```python
from build123d import *

# Parameters (mm, degrees)
SKETCH_8_R               = 2.25
EXTRUDE_23_DEPTH         = 6.3
EXTRUDE_24_DEPTH         = 3.8
CUT_EXTRUDE_START        = -2
SKETCH_8_5_R             = 1
CUT_EXTRUDE_2_DEPTH      = 9.8
PATTERN_CIRCULAR_1_COUNT = 3
CUT_EXTRUDE_3_DEPTH      = 3.7
PATTERN_CIRCULAR_2_COUNT = 3
CUT_EXTRUDE_6_DEPTH      = 1
SKETCH_12_W              = 12
SKETCH_12_H              = 8
SKETCH_12_W_2            = 11
SKETCH_12_H_2            = 7
EXTRUDE_1_DEPTH          = 3
SKETCH_14_R              = 6.2
SKETCH_14_R_2            = 4.5
CUT_EXTRUDE_7_DEPTH      = 1
FILLET_1_R               = 0.5


with BuildPart() as part:
    # 草图7 → 旋转1 (revolve)
    with BuildSketch(Plane.XY):
        Polygon((0, 0), (24.6, 0), (25.3, 7.8), (24.8, 7.8), (24.755128205, 7.3), (24.255128205, 7.3), (23.68974359, 1), (0, 1), align=None)
    revolve(axis=Axis((0, 1, 0), (0, -1, 0)))

    # 草图8 → 凸台-拉伸23 (add)
    with BuildSketch(Plane(origin=(0, 1, 0), x_dir=(1, 0, 0), z_dir=(0, 1, 0))):
        with Locations((0, 22.05)):
            Circle(SKETCH_8_R)
    extrude_23 = extrude(amount=EXTRUDE_23_DEPTH)

    # 草图8<4> → 凸台-拉伸24 (add)
    with BuildSketch(Plane(origin=(0, 1, 0), x_dir=(1, 0, 0), z_dir=(0, 1, 0))):
        with BuildLine():
            Line((-3, 22.05), (-3, 24.114103757))
            ThreePointArc((-3, 24.114103757), (0, 24.3), (3, 24.114103757))
            Line((3, 24.114103757), (3, 22.05))
            ThreePointArc((3, 22.05), (0, 19.05), (-3, 22.05))
        make_face()
    extrude_24 = extrude(amount=EXTRUDE_24_DEPTH)

    # 草图8<5> → 切除-拉伸2 (cut)
    with BuildSketch(Plane(origin=(0, 1, 0), x_dir=(1, 0, 0), z_dir=(0, 1, 0)).offset(CUT_EXTRUDE_START)):
        with Locations((0, 22.05)):
            Circle(SKETCH_8_5_R)
    cut_extrude_2 = extrude(amount=CUT_EXTRUDE_2_DEPTH, mode=Mode.SUBTRACT)

    # 阵列(圆周)1: 凸台-拉伸23, 凸台-拉伸24, 切除-拉伸2 ×3 about axis
    pattern_circular_1_axis = Axis((0, 0, 0), (0, 1, 0))
    for i in range(1, PATTERN_CIRCULAR_1_COUNT):
        add(extrude_23.rotate(pattern_circular_1_axis, i * 360 / PATTERN_CIRCULAR_1_COUNT))
        add(extrude_24.rotate(pattern_circular_1_axis, i * 360 / PATTERN_CIRCULAR_1_COUNT))
        add(cut_extrude_2.rotate(pattern_circular_1_axis, i * 360 / PATTERN_CIRCULAR_1_COUNT), mode=Mode.SUBTRACT)

    # 草图9 → 切除-拉伸3 (cut)
    with BuildSketch(Plane.XZ):
        with BuildLine():
            Line((2, -22.05), (2, -26.095171051))
            Line((2, -26.095171051), (-2, -26.095171051))
            Line((-2, -26.095171051), (-2, -22.05))
            ThreePointArc((-2, -22.05), (0, -20.05), (2, -22.05))
        make_face()
    cut_extrude_3 = extrude(amount=-CUT_EXTRUDE_3_DEPTH, mode=Mode.SUBTRACT)

    # 阵列(圆周)2: 切除-拉伸3 ×3 about axis
    pattern_circular_2_axis = Axis((0, 0, 0), (0, 1, 0))
    for i in range(1, PATTERN_CIRCULAR_2_COUNT):
        add(cut_extrude_3.rotate(pattern_circular_2_axis, i * 360 / PATTERN_CIRCULAR_2_COUNT), mode=Mode.SUBTRACT)

    # 草图11 → 切除-拉伸6 (cut)
    with BuildSketch(Plane(origin=(0, 1, 0), x_dir=(1, 0, 0), z_dir=(0, 1, 0))):
        Polygon((10, 15.975), (10, 4.975), (17.7, 4.975), (18.7, 5.975), (18.7, 14.975), (17.7, 15.975), align=None)
        Polygon((13.924175705, 3.975), (13.924175705, -7.025), (21.624175705, -7.025), (22.624175705, -6.025), (22.624175705, 2.975), (21.624175705, 3.975), align=None)
    extrude(amount=-CUT_EXTRUDE_6_DEPTH, mode=Mode.SUBTRACT)

    # 草图12 → 拉伸-薄壁1 (add)
    with BuildSketch(Plane(origin=(0, 1, 0), x_dir=(1, 0, 0), z_dir=(0, 1, 0))):
        with Locations((0, -16.8)):
            Rectangle(SKETCH_12_W, SKETCH_12_H)
        with Locations((0, -16.8)):
            Rectangle(SKETCH_12_W_2, SKETCH_12_H_2, mode=Mode.SUBTRACT)
    extrude(amount=EXTRUDE_1_DEPTH)

    # 草图14 → 切除-拉伸7 (cut)
    with BuildSketch(Plane(origin=(0, 1, 0), x_dir=(1, 0, 0), z_dir=(0, 1, 0))):
        Circle(SKETCH_14_R)
        with Locations((11.70765428, -15.20450888)):
            Circle(SKETCH_14_R_2)
    extrude(amount=-CUT_EXTRUDE_7_DEPTH, mode=Mode.SUBTRACT)

    # 圆角1
    fillet_1_edges = [part.edges().sort_by_distance(p)[0] for p in [
        (-21.304224933, 0, -12.3),
        (-2, 0, -23.284282198),
        (2, 0, -23.284282198),
        (0, 0, -20.05),
        (0, 0, 24.6),
        (18.088117647, 0, -16.67273223),
        (-19.164779892, 0, 13.374191906),
        (-21.164779892, 0, 9.910090291),
        (-17.363809346, 0, 10.025),
        (21.164779892, 0, 9.910090291),
        (19.164779892, 0, 13.374191906),
        (17.363809346, 0, 10.025),
    ]]
    fillet(fillet_1_edges, radius=FILLET_1_R)


solid = part.part
```
Verification items for the finished model (mm, model axes). A direction names the side the tool comes from. Give positions to 0.01 mm unless a question says otherwise; leave off trailing zeros. Order: outer loops, then holes, each group sorted by start corner. A loop starts at its lowest first (then second) coordinate and runs counter-clockwise, first axis right, second up. Notation, with made-up numbers: (32, 45.5) - (41, 45.5) arc R30 cw to (41, 73.5) - close; hole circle Ø11 at (-6, 57.25). An arc over 180 degrees is marked (long way). Answer as CSV lines item,"result". Start each with the question number.
Item 1: Gauge pin test, flat ends, axial feed: pin 1 (12 mm diameter, centred on x = 10, z = 11.5, fed in from +Y); pin 2 (3 mm diameter, centred on y = 1, z = 5.5, fed in from +X); pin 3 (1.5 mm diameter, centred on x = -19, z = 11, fed in from -Y); pin 4 (2 mm diameter, centred on x = 17, y = 4.5, fed in from -Z). Record the tip position at first contact, or that the pin passes through.
Item 2: Access from +Z, -Z, +X, -X, +Y, -Y to the whole of each face (thin tool, end or side, straight path). Record for faces 4 (the face through (18.3, 5.47, 11.63)), 5 (the face through (-19.33, 2.08, 13.47)), 6 (the face through (-21.292, 2.078, 9.984)), 7 (the face through (0, 2, 20.3)).
Item 3: Mould release check, pull along Z, two halves, no side actions. Record for faces 1 (the face through (-5.366, 1.731, -24.167)), 2 (the face through (2, 2, -23)), 3 (the face through (-17, 7.3, 11)): released by +Z, released by -Z, zero draft, split by the parting line, or undercut.
Item 4: Section check B-B, the plane y = 1.75. State how many separate pieces and enclosed holes the cut face has, plus the area to 3 significant figures.
Item 5: Section check A-A, the plane z = 0. Record the boundary of the cut face in (x, y).
Item 6: Material ranges on L1, parallel to X at y = 3, z = 20.5; L2, parallel to X at y = 1.25, z = -20; L3, parallel to Z at x = 1.5, y = 1.25, recorded low to high.
Filled in:
1,pin 1,"y = 4"
1,pin 2,"x = 24.4"
1,pin 3,"through"
1,pin 4,"z = -19.22"
2,face 4,"+Y, -Y"
2,face 5,"-X, -Y"
2,face 6,"-Y"
2,face 7,"+Y"
3,face 1,"split by the parting line"
3,face 2,"zero draft"
3,face 3,"undercut"
4,separate pieces,"2"
4,enclosed holes,"2"
4,area,"192 mm^2"
5,outline,"(-25.3, 7.8) - (-24.64, 0.46) arc R0.5 ccw to (-24.14, 0) - (-6.2, 0) - (-6.2, 1) - (-23.69, 1) - (-24.26, 7.3) - (-24.76, 7.3) - (-24.8, 7.8) - close; (6.2, 0) - (13.92, 0) - (13.92, 1) - (6.2, 1) - close; (22.62, 0) - (24.14, 0) arc R0.5 ccw to (24.64, 0.46) - (25.3, 7.8) - (24.8, 7.8) - (24.76, 7.3) - (24.26, 7.3) - (23.69, 1) - (22.62, 1) - close"
6,L1,"-14.08 to -12.23, -6 to 6, 12.23 to 14.08"
6,L2,"-14.52 to -12.74, -2.19 to 2.19, 12.74 to 14.52"
6,L3,"-20.73 to -19.45, 12.8 to 13.3, 20.3 to 20.8, 23.66 to 24.67"
